For this review, take the finished solid that the model builds, in its own axes (mm). Coordinates: 2 decimals unless noted, no trailing zeros. Write each loop counter-clockwise with the first axis right and the second up, starting at its lowest first coordinate (ties: lowest second). Pieces come first, ordered by that corner, then holes. Notation, with made-up numbers: M 68.5,-10 L 105.5,-10 A13 ccw 105.5,0 Z; hole C -31,-15.75 d3. An arc over 180 degrees is marked long. Return JSON: item names as keys, results as strings.
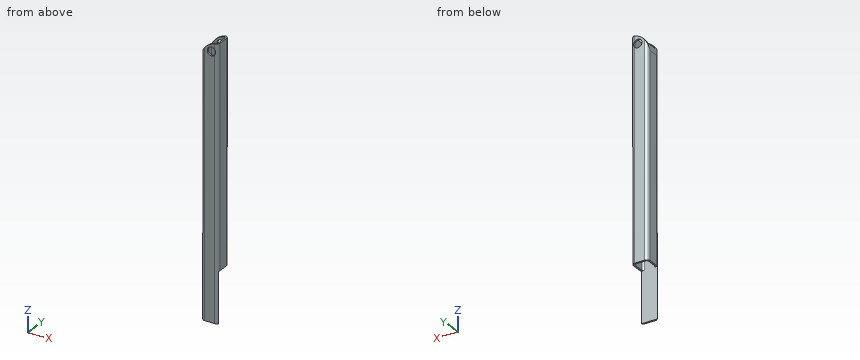
```python
from build123d import *

# Parameters (mm, degrees)
BOSS_EXTRUDE1_DEPTH = 203.2
SKETCH2_R           = 3.175
CUT_EXTRUDE1_DEPTH  = 13.7
SKETCH3_W           = 38.1
SKETCH3_H           = 11.43
CUT_EXTRUDE2_DEPTH  = 13.7000001
CUT_EXTRUDE3_DEPTH  = 13.7000001


with BuildPart() as part:
    # Sketch1 → Boss-Extrude1 (new body)
    with BuildSketch(Plane.XY):
        with BuildLine():
            Line((2.54, 0), (10.16, 0))
            ThreePointArc((10.16, 0), (11.956051224, 0.743948776), (12.7, 2.54))
            Line((12.7, 2.54), (12.7, 10.16))
            ThreePointArc((12.7, 10.16), (11.956051224, 11.956051224), (10.16, 12.7))
            Line((10.16, 12.7), (2.54, 12.7))
            ThreePointArc((2.54, 12.7), (0.743948776, 11.956051224), (0, 10.16))
            Line((0, 10.16), (0, 2.54))
            ThreePointArc((0, 2.54), (0.743948776, 0.743948776), (2.54, 0))
        make_face()
        with BuildLine():
            Line((2.54, 1.27), (10.16, 1.27))
            ThreePointArc((10.16, 1.27), (11.058025612, 1.641974388), (11.43, 2.54))
            Line((11.43, 2.54), (11.43, 10.16))
            ThreePointArc((11.43, 10.16), (11.058025612, 11.058025612), (10.16, 11.43))
            Line((10.16, 11.43), (2.54, 11.43))
            ThreePointArc((2.54, 11.43), (1.641974388, 11.058025612), (1.27, 10.16))
            Line((1.27, 10.16), (1.27, 2.54))
            ThreePointArc((1.27, 2.54), (1.641974388, 1.641974388), (2.54, 1.27))
        make_face(mode=Mode.SUBTRACT)
    extrude(amount=BOSS_EXTRUDE1_DEPTH)

    # Sketch2 → Cut-Extrude1 (cut, through all)
    with BuildSketch(Plane(origin=(0, 12.7, 0), x_dir=(1, 0, 0), z_dir=(0, 1, 0))):
        with Locations((7.747, -196.85)):
            Circle(SKETCH2_R)
    extrude(amount=-CUT_EXTRUDE1_DEPTH, mode=Mode.SUBTRACT)

    # Sketch3 → Cut-Extrude2 (cut, through all)
    with BuildSketch(Plane.ZY):
        with Locations((19.05, 6.985)):
            Rectangle(SKETCH3_W, SKETCH3_H)
    extrude(amount=-CUT_EXTRUDE2_DEPTH, mode=Mode.SUBTRACT)

    # Sketch4 → Cut-Extrude3 (cut, through all)
    with BuildSketch(Plane(origin=(0, 12.7, 0), x_dir=(1, 0, 0), z_dir=(0, 1, 0))):
        with BuildLine():
            Line((0, -203.2), (12.7, -203.2))
            ThreePointArc((12.7, -203.2), (3.719743879, -199.480256121), (0, -190.5))
            Line((0, -190.5), (0, -203.2))
        make_face()
    extrude(amount=-CUT_EXTRUDE3_DEPTH, mode=Mode.SUBTRACT)


solid = part.part
```
1. We need section A-A (y = 4.25). State the section outline as (x, z) points, plus the area to 3 significant figures.
Checks:
{"outline": "M 0,38.1 L 1.27,38.1 L 1.27,196.04 A12.7 ccw 0,190.5 Z; M 11.43,38.1 L 12.7,38.1 L 12.7,203.2 A12.7 ccw 11.43,203.14 Z", "area": "408 mm2"}
2. We need section C-C (x = 8.25). State the section outline as (y, z) points.
Checks:
{"outline": "M 0,0 L 1.27,0 L 1.27,193.72 L 0,193.72 Z; M 0,199.98 L 1.27,199.98 L 1.27,202.39 L 0,202.39 Z; M 11.43,38.1 L 12.7,38.1 L 12.7,193.72 L 11.43,193.72 Z; M 11.43,199.98 L 12.7,199.98 L 12.7,202.39 L 11.43,202.39 Z"}
3. Wall thickness on L1, parallel to Y at x = 3, z = 53; L2, parallel to Z at x = 8.25, y = 11.5: over which ranges is each line inside the solid? List them lowest first. Write a range as from..to.
Checks:
{"L1": "0..1.27, 11.43..12.7", "L2": "38.1..193.72, 199.98..202.39"}
4. We need section B-B (z = 43). State the section outline as (x, y) points.
Checks:
{"outline": "M 0,2.54 A2.54 ccw 2.54,0 L 10.16,0 A2.54 ccw 12.7,2.54 L 12.7,10.16 A2.54 ccw 10.16,12.7 L 2.54,12.7 A2.54 ccw 0,10.16 Z; hole M 1.27,2.54 A1.27 ccw 2.54,1.27 L 10.16,1.27 A1.27 ccw 11.43,2.54 L 11.43,10.16 A1.27 ccw 10.16,11.43 L 2.54,11.43 A1.27 ccw 1.27,10.16 Z"}
5. Clearance check with flat-ended pins moving along their axes: pin 1 Ø4 at (x, y) = (9.5, 7.5) entering from +Z; pin 2 Ø2 at (x, y) = (10, 10.5) entering from -Z. State where each tip first meets the part, or that it passes through.
Checks:
{"pin 1": "z = 203.14", "pin 2": "z = 38.1"}
